from build123d import *

# Parameters (mm, degrees)
EXTRUDE_1_DEPTH     = 240
SKETCH_3_R          = 1
CUT_EXTRUDE_1_DEPTH = 31
SKETCH_4_R          = 1
CUT_EXTRUDE_2_DEPTH = 31


with BuildPart() as part:
    # 草图1 → 凸台-拉伸1 (new body, symmetric)
    with BuildSketch(Plane(origin=(0, 0, 0), x_dir=(1, 0, 0), z_dir=(0, 1, 0))):
        Polygon((14.142135624, 0), (0, 14.142135624), (-14.142135624, 0), (0, -14.142135624), align=None)
        Polygon((12.727922061, 0), (0, 12.727922061), (-12.727922061, 0), (0, -12.727922061), align=None, mode=Mode.SUBTRACT)
    extrude(amount=EXTRUDE_1_DEPTH, both=True)

    # 草图3 → 切除-拉伸1 (cut, through all)
    with BuildSketch(Plane(origin=(7.071067812, 0, 7.071067812), x_dir=(0.707106781, 0, -0.707106781), z_dir=(0.707106781, 0, 0.707106781))):
        with Locations((0, 230)):
            Circle(SKETCH_3_R)
        with Locations((0, 190)):
            Circle(SKETCH_3_R)
        with Locations((0, -190)):
            Circle(SKETCH_3_R)
        with Locations((0, -230)):
            Circle(SKETCH_3_R)
    extrude(amount=-CUT_EXTRUDE_1_DEPTH, mode=Mode.SUBTRACT)

    # 草图4 → 切除-拉伸2 (cut, through all)
    with BuildSketch(Plane(origin=(7.071067812, 0, 7.071067812), x_dir=(0.707106781, 0, -0.707106781), z_dir=(0.707106781, 0, 0.707106781))):
        with Locations((0, 100)):
            Circle(SKETCH_4_R)
        Circle(SKETCH_4_R)
        with Locations((0, -100)):
            Circle(SKETCH_4_R)
    extrude(amount=-CUT_EXTRUDE_2_DEPTH, mode=Mode.SUBTRACT)


solid = part.part
The listing builds one solid part. Answer for the finished solid, in the listing's coordinates (mm). A direction names the side the tool comes from. Coordinates: 2 decimals unless noted, no trailing zeros. Loops run counter-clockwise (first coordinate to the right, second up) from the corner with the lowest first, then second, coordinate; pieces in that order, holes last. Notation, with made-up numbers: (17, 51.5) -> (22, 51.5) arc R28 ccw to (22, 88.5) -> close; hole circle Ø10 at (-20, -27). An arc over 180 degrees is marked (long way). Write item = value, one per line. Start each with the question number.
1) A cutting plane is placed at A-A (y = 63). Give the vertices of the cut face in (x, z), then the cut area to 3 significant figures.
2) A tool of negligible diameter and unlimited length cuts with its end or side. For faces 1 (the face through (-6.275, 3.36, -6.453)), 2 (the face through (7.17, 3.36, -6.97)), from which of +Z, -Z, +X, -X, +Y, -Y can it reach the whole face along a straight path? Write none if from no direction.
3) The mould has two halves that part along X. Classify faces 3 (the face through (-7.17, 3.36, 6.97)), 4 (the face through (6.453, 3.36, -6.275)), 5 (the face through (-7, -240, -6)), 6 (the face through (6.97, 3.36, 7.17)): released by +X, released by -X, zero draft, split by the parting line, or undercut.
4) Given pin 1 Ø1.5 at (x, y) = (-9, 171.5) entering from +Z; pin 2 Ø6 at (x, y) = (-7.5, -18.5) entering from -Z; pin 3 Ø12 at (y, z) = (127, 7.5) entering from -X, each flat-ended and moving along its own axis, determine where each tip first touches the part or whether it passes through.
5) Straight lines are drawn through the part: line 1 (Z direction, x = 0, y = 83); line 2 (X direction, y = -117, z = 4.5); line 3 (X direction, y = 38.5, z = -3.5). For each, find the intervals that lie inside material, in ascending order. Write a range as from..to.
Responses:
q1.outline = (-14.14, 0) -> (0, -14.14) -> (14.14, 0) -> (0, 14.14) -> close; hole (-12.73, 0) -> (0, -12.73) -> (12.73, 0) -> (0, 12.73) -> close
q1.area = 76.0 mm²
q2.face_1 = +Y, -Y
q2.face_2 = -Z, +X, +Y, -Y
q3.face_3 = released by -X
q3.face_4 = undercut
q3.face_5 = zero draft
q3.face_6 = released by +X
q4.pin_1 = 5.89
q4.pin_2 = -9.64
q4.pin_3 = -12.64
q5.line_1 = -14.14..-12.73, 12.73..14.14
q5.line_2 = -9.64..-8.23, 8.23..9.64
q5.line_3 = -10.64..-9.23, 9.23..10.64
